Read the model definition and answer for the solid it produces. Units are mm, in the model's axes. A direction names the side the tool comes from. Round coordinates to 2 decimals unless told otherwise and drop trailing zeros. Order: outer loops, then holes, each group sorted by start corner. A loop starts at its lowest first (then second) coordinate and runs counter-clockwise, first axis right, second up. Notation, with made-up numbers: (34, -5.75) -> (50, -5.75) arc R17 cw to (50, 14.25) -> close; hole circle Ø1 at (14.5, 11.5). An arc over 180 degrees is marked (long way). Use a Markdown table: item, result. Add a question column.
1. Section A-A, the plane y = -1.9 is taken. Give the number of separate pieces and of enclosed holes in the cut face, then the cut area to 3 significant figures.
2. The mould has two halves that part along X. Classify faces 1 (the face through (0.193, -1.503, 123.823)), 2 (the face through (41.28, -1.5, 0.14)), 3 (the face through (-12.556, -1.503, 90.838)): +X half, -X half, draft (parallel to the pull), parting line (faces both ways), or undercut.
3. Consider L1, parallel to Z at x = 31.5, y = -0.25; L2, parallel to X at y = -1.2, z = 94.5; L3, parallel to Z at x = 43, y = -1.25. Determine where each line is inside the solid, lowest interval first. Write a range as [from, to].
4. Given pin 1 (1.5 mm diameter, centred on x = 36.5, y = -1, fed in from +Z); pin 2 (1 mm diameter, centred on x = -1.5, y = -0.5, fed in from -Z), each flat-ended and moving along its own axis, determine where each tip first touches the part or whether it passes through.
5. Section C-C, the plane x = 25.5 is taken. Give the vertices of the cut face in (y, z), then the cut area to 3 significant figures.
6. Section D-D, the plane z = 37 is taken. Give the vertices of the cut face in (x, y), then the cut area to 3 significant figures.
7. Section B-B, the plane x = 43 is taken. Give the vertices of the cut face in (y, z), then the cut area to 3 significant figures.
8. For faces 4 (the face through (12.9, -1.5, 38.9)), 5 (the face through (-0.69, -1.5, -3.1)), 6 (the face through (31, -2, 7.938)), determine the directions among +Z, -Z, +X, -X, +Y, -Y from which every point of the face is accessible in a straight line to the end or side of a thin tool.
```python
from build123d import *

# Parameters (mm, degrees)
F0_R     = 3.175
F1_DEPTH = 3.048


with BuildPart() as f1:
    # F0 (on Front) → F1 (new body)
    with BuildSketch(Plane.XZ):
        with BuildLine():
            ThreePointArc((9.450293, 115.490625), (0, 123.825), (-9.450293, 115.490625))
            ThreePointArc((-9.450293, 115.490625), (-0.596483, 104.793695), (9.525, 114.3))
            ThreePointArc((9.525, 114.3), (9.506305, 114.896483), (9.450293, 115.490625))
        make_face()
        with Locations((0, 114.3)):
            Circle(F0_R, mode=Mode.SUBTRACT)
        with BuildLine():
            Line((-9.450293, 115.490625), (-15.750488, 65.484375))
            ThreePointArc((-15.750488, 65.484375), (0, 79.375), (15.750488, 65.484375))
            Line((15.750488, 65.484375), (9.450293, 115.490625))
            ThreePointArc((9.450293, 115.490625), (9.506305, 114.896483), (9.525, 114.3))
            ThreePointArc((9.525, 114.3), (-0.596483, 104.793695), (-9.450293, 115.490625))
        make_face()
        with Locations((-3.175, 95.25)):
            Circle(F0_R, mode=Mode.SUBTRACT)
        with BuildLine():
            ThreePointArc((-15.750488, 65.484375), (-15.875, 63.5), (-15.750488, 61.515625))
            ThreePointArc((-15.750488, 61.515625), (0, 47.625), (15.750488, 61.515625))
            ThreePointArc((15.750488, 61.515625), (15.843841, 62.505861), (15.875, 63.5))
            ThreePointArc((15.875, 63.5), (15.843841, 64.494139), (15.750488, 65.484375))
            ThreePointArc((15.750488, 65.484375), (0, 79.375), (-15.750488, 65.484375))
        make_face()
        with Locations((0, 63.5)):
            Circle(F0_R, mode=Mode.SUBTRACT)
        with BuildLine():
            ThreePointArc((-7.875244, -0.992188), (-0.497069, 7.921921), (7.9375, 0))
            ThreePointArc((7.9375, 0), (5.61266, -5.61266), (0, -7.9375))
            Line((0, -7.9375), (44.45, -7.9375))
            ThreePointArc((44.45, -7.9375), (36.5125, 0), (44.45, 7.9375))
            Line((44.45, 7.9375), (18.014958, 7.9375))
            ThreePointArc((18.014958, 7.9375), (12.052308, 10.629137), (10.127114, 16.881475))
            Line((10.127114, 16.881475), (15.750488, 61.515625))
            ThreePointArc((15.750488, 61.515625), (0, 47.625), (-15.750488, 61.515625))
            Line((-15.750488, 61.515625), (-7.875244, -0.992188))
        make_face()
        with BuildLine():
            ThreePointArc((0, -7.9375), (5.61266, -5.61266), (7.9375, 0))
            ThreePointArc((7.9375, 0), (-0.497069, 7.921921), (-7.875244, -0.992188))
            ThreePointArc((-7.875244, -0.992188), (-5.250163, -5.953125), (0, -7.9375))
        make_face()
        Circle(F0_R, mode=Mode.SUBTRACT)
        with BuildLine():
            ThreePointArc((44.45, 7.9375), (36.5125, 0), (44.45, -7.9375))
            ThreePointArc((44.45, -7.9375), (50.06266, -5.61266), (52.3875, 0))
            ThreePointArc((52.3875, 0), (50.06266, 5.61266), (44.45, 7.9375))
        make_face()
        with Locations((44.45, 0)):
            Circle(F0_R, mode=Mode.SUBTRACT)
    extrude(amount=F1_DEPTH)


solid = f1.part
```
Verdict:
| question | item | result |
|---|---|---|
| 1 | separate pieces | 1 |
| 1 | enclosed holes | 5 |
| 1 | area | 3,610 mm2 |
| 2 | face 1 | parting line |
| 2 | face 2 | undercut |
| 2 | face 3 | -X half |
| 3 | L1 | z = [-7.94, 7.94] |
| 3 | L2 | x = [-12.09, -6.26], [-0.09, 12.09] |
| 3 | L3 | z = [-7.94, -2.82], [2.82, 7.94] |
| 4 | pin 1 | stops at z = 7.94 |
| 4 | pin 2 | stops at z = -7.87 |
| 5 | outline | (-3.05, -7.94) -> (0, -7.94) -> (0, 7.94) -> (-3.05, 7.94) -> close |
| 5 | area | 48.4 mm2 |
| 6 | outline | (-12.66, -3.05) -> (12.66, -3.05) -> (12.66, 0) -> (-12.66, 0) -> close |
| 6 | area | 77.2 mm2 |
| 7 | outline | (-3.05, -7.94) -> (0, -7.94) -> (0, -2.82) -> (-3.05, -2.82) -> close; (-3.05, 2.82) -> (0, 2.82) -> (0, 7.94) -> (-3.05, 7.94) -> close |
| 7 | area | 31.2 mm2 |
| 8 | face 4 | +X, +Y, -Y |
| 8 | face 5 | +Y, -Y |
| 8 | face 6 | +Z, +X, +Y, -Y |
